from build123d import *

# Parameters (mm, degrees)
SKETCH1_R           = 5.461
BOSS_EXTRUDE1_DEPTH = 25.4
SKETCH2_R           = 4.191
CUT_EXTRUDE1_DEPTH  = 7.62
SKETCH3_R           = 5.461
BOSS_EXTRUDE2_DEPTH = 50.8
REVOLVE2_ANGLE      = 90
SKETCH8_R           = 2.7305
SKETCH9_R           = 2.7305
BOSS_EXTRUDE3_DEPTH = 7.62
REVOLVE3_ANGLE      = 180


with BuildPart() as part:
    # Sketch1 → Boss-Extrude1 (new body)
    with BuildSketch(Plane(origin=(0, 0, 0), x_dir=(0, 0, -1), z_dir=(1, 0, 0))):
        Circle(SKETCH1_R)
    extrude(amount=BOSS_EXTRUDE1_DEPTH)

    # Sketch2 → Cut-Extrude1 (cut)
    with BuildSketch(Plane.ZY):
        Circle(SKETCH2_R)
    extrude(amount=-CUT_EXTRUDE1_DEPTH, mode=Mode.SUBTRACT)

    # Sketch3 → Boss-Extrude2 (add)
    with BuildSketch(Plane(origin=(0, 0, 0), x_dir=(1, 0, 0), z_dir=(0, 1, 0))):
        with Locations((25.4, 0)):
            Circle(SKETCH3_R)
    extrude(amount=BOSS_EXTRUDE2_DEPTH)

    # Sketch7 → Revolve2 (revolve)
    with BuildSketch(Plane(origin=(25.4, 0, 0), x_dir=(0, 0, -1), z_dir=(1, 0, 0))):
        with BuildLine():
            Line((5.461, 0), (-5.461, 0))
            ThreePointArc((-5.461, 0), (0, -5.461), (5.461, 0))
        make_face()
    revolve(axis=Axis((25.4, 0, -5.461), (0, 0, 1)), revolution_arc=REVOLVE2_ANGLE)

    # Sketch8 → section 1 of loft2
    with BuildSketch(Plane(origin=(0, 152.4, 0), x_dir=(1, 0, 0), z_dir=(0, 1, 0)), mode=Mode.PRIVATE) as loft2_s1:
        with Locations((25.4, 0)):
            Circle(SKETCH8_R)
    # loft from a face of the part (loft2)
    loft([part.faces().sort_by_distance((25.4, 50.8, 0))[0], loft2_s1.sketch])

    # Sketch9 → Boss-Extrude3 (add)
    with BuildSketch(Plane(origin=(0, 152.4, 0), x_dir=(1, 0, 0), z_dir=(0, 1, 0))):
        with Locations((25.4, 0)):
            Circle(SKETCH9_R)
    extrude(amount=BOSS_EXTRUDE3_DEPTH)

    # Sketch10 → Revolve3 (revolve)
    with BuildSketch(Plane(origin=(0, 160.02, 0), x_dir=(1, 0, 0), z_dir=(0, 1, 0))):
        with BuildLine():
            Line((25.4, 2.7305), (25.4, -2.7305))
            ThreePointArc((25.4, -2.7305), (28.1305, 0), (25.4, 2.7305))
        make_face()
    revolve(axis=Axis((25.4, 160.02, -2.7305), (0, 0, 1)), revolution_arc=REVOLVE3_ANGLE)


solid = part.part
The listing builds one solid part. Answer for the finished solid, in the listing's coordinates (mm). A direction names the side the tool comes from. Round coordinates to 2 decimals unless told otherwise and drop trailing zeros. Order: outer loops, then holes, each group sorted by start corner. A loop starts at its lowest first (then second) coordinate and runs counter-clockwise, first axis right, second up. Notation, with made-up numbers: (40, 14.5) -> (79, 14.5) arc R19 ccw to (79, 27.5) -> close; hole circle Ø11 at (3, -2). An arc over 180 degrees is marked (long way). Put each result on its own line as item: value.
Q1. Consider line 1 along Y through (x, z) = (4, 0); line 2 along Y through (x, z) = (4.5, 2); line 3 along Y through (x, z) = (13, 0.25). Determine where each line is inside the solid, lowest interval first.
Results list:
line 1: -5.46 to -4.19, 4.19 to 5.46
line 2: -5.08 to -3.68, 3.68 to 5.08
line 3: -5.46 to 5.46
Q2. Which of the six approach directions +Z, -Z, +X, -X, +Y, -Y give full straight-line access (tool end or side, diameter ignored) to faces 4 (the flat face through (7.62, 0, 0)), 5 (the flat face through (0, -4, -2)), 6 (the cylindrical face through (22.672, 156.157, -0.12))?
Results list:
face 4: -X
face 5: +Z, -Z, -X, +Y, -Y
face 6: +Y
Q3. Each of these flat-tipped pins is pushed along its axis until it touches: P1, Ø4, axis at y = 96.5, z = -4, coming from the -X side; P2, Ø1, axis at x = 27, z = 0, coming from the +Y side; P3, Ø5, axis at x = 8, z = 2, coming from the +Y side. Where does it stop, or does it pass through?
Results list:
P1: x = 21.67
P2: y = 162.52
P3: y = 5.46
Q4. Section B-B, the plane x = 10 is taken. Write down the section's boundary in (y, z).
Results list:
outline: circle Ø10.92 at (0, 0)
Q5. Determine the mould class of faces 1 (the cylindrical face through (12.52, -5.33, 1.18)), 2 (the cylindrical face through (3.757, 1.259, 3.997)), 3 (the cylindrical face through (30.445, 25.044, 2.092)) for opening direction Y: pulls with the +Y half, pulls with the -Y half, needs draft (parallel to the pull), parting line crosses it, or undercut.
Results list:
face 1: parting line crosses it
face 2: undercut
face 3: needs draft
Q6. Section A-A, the plane y = 54.5 is taken. Write down the section's boundary in (x, z), and give its area (3 significant figures).
Results list:
outline: circle Ø10.72 at (25.4, 0)
area: 90.3 mm^2
